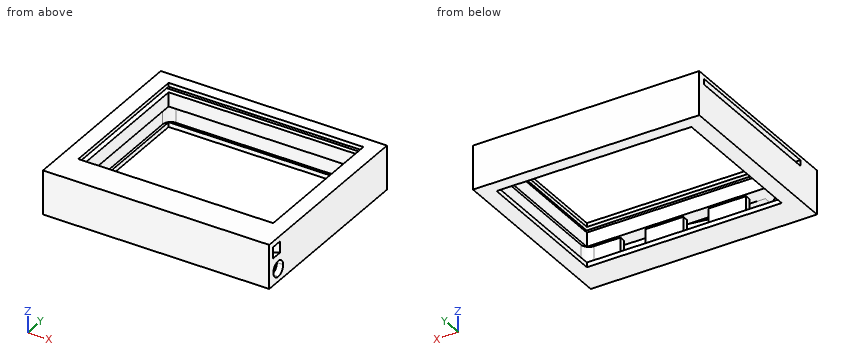
```python
from build123d import *

# Parameters (mm, degrees)
F0_W      = 180
F0_H      = 150
F0_W_2    = 155
F0_H_2    = 115
F1_DEPTH  = 35
F2_W      = 122.5
F2_H      = 4.5
F3_DEPTH  = 170
F5_W      = 159
F5_H      = 119
F6_DEPTH  = 6.25
F7_R      = 6.5
F9_DEPTH  = 6.25
F11_DEPTH = 9
F12_R     = 25
F14_DEPTH = 5
F15_W     = 20
F15_H     = 12.5
F16_DEPTH = 4.5


with BuildPart() as f1:
    # F0 (on Top) → F1 (new body)
    with BuildSketch(Plane.XY):
        with Locations((90, 75)):
            Rectangle(F0_W, F0_H)
        with Locations((90, 82.5)):
            Rectangle(F0_W_2, F0_H_2, mode=Mode.SUBTRACT)
    extrude(amount=F1_DEPTH)

    # F2 (on face) → F3 (cut)
    with BuildSketch(Plane(origin=(0, 0, 0), x_dir=(0, -1, 0), z_dir=(-1, 0, 0))):
        with Locations((-82.5, 29.75)):
            Rectangle(F2_W, F2_H)
    extrude(amount=-F3_DEPTH, mode=Mode.SUBTRACT)

    # F5 (on offset) → F6 (cut, symmetric)
    with BuildSketch(Plane(origin=(0, 0, 10), x_dir=(1, 0, 0), z_dir=(0, 0, -1))):
        with Locations((90, -82.5)):
            Rectangle(F5_W, F5_H)
    extrude(amount=F6_DEPTH, both=True, mode=Mode.SUBTRACT)

    # F7
    f7_edges = [f1.edges().sort_by_distance(p)[0] for p in [
        (169.5, 142, 10),
        (10.5, 142, 10),
        (10.5, 23, 10),
        (169.5, 23, 10),
    ]]
    fillet(f7_edges, radius=F7_R)

    # F8 (on offset) → F9 (cut, symmetric)
    with BuildSketch(Plane(origin=(0, 0, 10), x_dir=(1, 0, 0), z_dir=(0, 0, -1))):
        with BuildLine():
            Line((32.8076118446, -4.5), (12.4038059223, -24.9038059223))
            ThreePointArc((12.4038059223, -24.9038059223), (14.5125576896, -23.4947830387), (17, -23))
            Line((17, -23), (42, -23))
            Line((42, -23), (42, -18.5))
            Line((42, -18.5), (180, -18.5))
            Line((180, -18.5), (180, -4.5))
            Line((180, -4.5), (32.8076118446, -4.5))
        make_face()
    extrude(amount=F9_DEPTH, both=True, mode=Mode.SUBTRACT)

    # F10 (on face) → F11 (cut)
    with BuildSketch(Plane(origin=(0, 4.5, 0), x_dir=(-1, 0, 0), z_dir=(0, 1, 0))):
        Polygon((-160, 16.25), (-125.2266702536, 16.25), (-32.8076118446, 16.25), (-180, 30.6089838486), (-180, 21.6089838486), align=None)
    extrude(amount=F11_DEPTH, mode=Mode.SUBTRACT)

    # F12
    f12_edges = [f1.edges().sort_by_distance(p)[0] for p in [
        (32.807612, 4.5, 10),
    ]]
    fillet(f12_edges, radius=F12_R)

    # F13 (on face) → F14 (join)
    with BuildSketch(Plane.YZ.offset(180)):
        with BuildLine():
            ThreePointArc((11.5, 16.25), (15.9194173824, 14.4194173824), (17.75, 10))
            ThreePointArc((17.75, 10), (15.9194173824, 5.5805826176), (11.5, 3.75))
            Line((11.5, 3.75), (18.5, 3.75))
            Line((18.5, 3.75), (18.5, 16.25))
            Line((18.5, 16.25), (11.5, 16.25))
        make_face()
        with BuildLine():
            ThreePointArc((11.5, 3.75), (5.25, 10), (11.5, 16.25))
            Line((11.5, 16.25), (4.5, 16.25))
            Line((4.5, 16.25), (4.5, 3.75))
            Line((4.5, 3.75), (11.5, 3.75))
        make_face()
    extrude(amount=-F14_DEPTH)

    # F15 (on face) → F16 (cut, through all)
    with BuildSketch(Plane(origin=(0, 23, 0), x_dir=(-1, 0, 0), z_dir=(0, 1, 0))):
        with Locations((-132, 10)):
            Rectangle(F15_W, F15_H)
        with Locations((-82, 10)):
            Rectangle(F15_W, F15_H)
    extrude(amount=-F16_DEPTH, mode=Mode.SUBTRACT)


solid = f1.part
```
Work out the finished part from the listing and answer in its coordinate system (mm). Coordinates: 2 decimals unless noted, no trailing zeros. Loops run counter-clockwise (first coordinate to the right, second up) from the corner with the lowest first, then second, coordinate; pieces in that order, holes last.
1) Consider probe 1 along Y at (x, z) = (100, 17); probe 2 along X at (y, z) = (67.5, 22.5); probe 3 along Y at (x, z) = (65, 11). Determine where each line is inside the solid, lowest interval first.
Results:
probe 1: y = 0 to 4.5, 13.5 to 25, 140 to 150
probe 2: x = 0 to 12.5, 167.5 to 180
probe 3: y = 0 to 4.5, 18.5 to 23, 142 to 150
2) Section B-B (y = 75) is taken. Give the vertices of the cut face in (x, z), plus the area to 4 significant figures.
Results:
outline: (0, 0) - (12.5, 0) - (12.5, 3.75) - (10.5, 3.75) - (10.5, 16.25) - (12.5, 16.25) - (12.5, 27.5) - (0, 27.5) - close; (0, 32) - (12.5, 32) - (12.5, 35) - (0, 35) - close; (167.5, 0) - (180, 0) - (180, 35) - (167.5, 35) - (167.5, 32) - (170, 32) - (170, 27.5) - (167.5, 27.5) - (167.5, 16.25) - (169.5, 16.25) - (169.5, 3.75) - (167.5, 3.75) - close
area: 757.5 mm2
3) Flat-ended cylindrical pins translate along their axes: pin 1 (1 mm diameter, centred on y = 16, z = 7.5, fed in from +X); pin 2 (10 mm diameter, centred on x = 158.5, y = 80, fed in from -Z). Find the tip coordinate at first contact, or state that the pin passes through.
Results:
pin 1: stops at x = 21.81
pin 2: passes through
4) Section A-A (x = 165.5) is taken. Give the number of separate pieces and of enclosed holes in the cut face, plus the area to 3 significant figures.
Results:
separate pieces: 2
enclosed holes: 2
area: 876 mm2
